Input: part model. Units: mm. Frame: model coordinates. A direction names the side the tool comes from. Round coordinates to 2 decimals unless told otherwise and drop trailing zeros. Loops run counter-clockwise (first coordinate to the right, second up) from the corner with the lowest first, then second, coordinate; pieces in that order, holes last. Notation, with made-up numbers: M 49,-13.5 L 73,-13.5 A25 cw 73,-1.5 Z; hole C -8.75,-31.75 d8. An arc over 180 degrees is marked long. Return JSON: item names as keys, results as strings. Group by question number.
1) Contact query for flat-ended pins moving along their axis: P1, Ø4, axis at x = 79, y = -17, coming from the +Z side; P2, Ø9, axis at x = -4.5, y = -15.5, coming from the -Z side; P3, Ø6.5, axis at x = -4.5, y = -19.5, coming from the +Z side; P4, Ø9.5, axis at y = -16.5, z = 15, coming from the +X side. Output: stop coordinate, or through.
2) Access query for faces 1 (the face through (12.5, -12, 71)), 2 (the face through (21, -12, -17)), 3 (the face through (21, -19.3, -2.5)), 4 (the face through (-21, -12, 17)). Directions: +Z, -Z, +X, -X, +Y, -Y. A direction counts if a zero-diameter tool reaches every point of the face in a straight line with its end or side. Return the directions, or none.
3) Section A-A (x = 0). Count the separate pieces of the cut face and the enclosed holes in it, plus the area to 3 significant figures.
4) Material intervals for line 1 (Z direction, x = 19.45, y = -14.5); line 2 (X direction, y = -18, z = 77); line 3 (Z direction, x = 122.65, y = -14.5), sorted ascending. Write a range as from..to.
5) Mould query, pull axis Z, two halves, no side actions, for faces 5 (the face through (1.08, -9.62, -18.46)), 6 (the face through (-73, -12, -12.5)), 7 (the face through (16, -20, 0)). Classes: +Z half, -Z half, draft (parallel to the pull), parting line (faces both ways), or undercut.
6) Section C-C (z = 82). Output: boundary loops of the cut face in (x, y), plus the area to 3 significant figures.
from build123d import *

# Parameters (mm, degrees)
F0_W      = 42
F0_H      = 42
F0_W_2    = 32
F0_H_2    = 32
F5_DEPTH  = 25
F1_W      = 25
F1_H      = 102
F2_W      = 102
F2_H      = 25
F3_W      = 102
F3_H      = 25
F4_W      = 25
F4_H      = 102
F6_DEPTH  = 25
F7_W      = 32
F7_H      = 32
F8_DEPTH  = 18
F9_W      = 100
F9_H      = 21
F10_DEPTH = 21
F11_W     = 100
F11_H     = 21
F12_DEPTH = 21
F13_W     = 21
F13_H     = 100
F14_DEPTH = 21
F15_W     = 21
F15_H     = 100
F16_DEPTH = 21
F18_D     = 10
F18_DEPTH = 11
F20_D     = 10
F20_DEPTH = 11
F22_D     = 10
F22_DEPTH = 11
F24_D     = 10
F24_DEPTH = 11
F26_D     = 20.9
F26_DEPTH = 3
F28_D     = 20.9
F28_DEPTH = 3
F30_D     = 20.9
F30_DEPTH = 3
F32_D     = 20.9
F32_DEPTH = 3


with BuildPart() as f5:
    # F0 (on Front) → F5 (new body)
    with BuildSketch(Plane.XZ):
        Rectangle(F0_W, F0_H)
        Rectangle(F0_W_2, F0_H_2, mode=Mode.SUBTRACT)
        Rectangle(F0_W_2, F0_H_2)
    extrude(amount=F5_DEPTH)

    # F1 (on Front) + F2 (on Front) + F3 (on Front) + F4 (on Front) → F6 (join)
    with BuildSketch(Plane.XZ):
        with Locations((0, -72)):
            Rectangle(F1_W, F1_H)
    with BuildSketch(Plane.XZ):
        with Locations((-72, 0)):
            Rectangle(F2_W, F2_H)
    with BuildSketch(Plane.XZ):
        with Locations((72, 0)):
            Rectangle(F3_W, F3_H)
    with BuildSketch(Plane.XZ):
        with Locations((0, 72)):
            Rectangle(F4_W, F4_H)
    extrude(amount=F6_DEPTH)

    # F7 (on face) → F8 (cut)
    with BuildSketch(Plane.XZ.offset(25)):
        Rectangle(F7_W, F7_H)
    extrude(amount=-F8_DEPTH, mode=Mode.SUBTRACT)

    # F9 (on face) → F10 (cut)
    with BuildSketch(Plane.XZ.offset(25)):
        with Locations((-71, 0)):
            Rectangle(F9_W, F9_H)
    extrude(amount=-F10_DEPTH, mode=Mode.SUBTRACT)

    # F11 (on face) → F12 (cut)
    with BuildSketch(Plane.XZ.offset(25)):
        with Locations((71, 0)):
            Rectangle(F11_W, F11_H)
    extrude(amount=-F12_DEPTH, mode=Mode.SUBTRACT)

    # F13 (on face) → F14 (cut)
    with BuildSketch(Plane.XZ.offset(25)):
        with Locations((0, 71)):
            Rectangle(F13_W, F13_H)
    extrude(amount=-F14_DEPTH, mode=Mode.SUBTRACT)

    # F15 (on face) → F16 (cut)
    with BuildSketch(Plane.XZ.offset(25)):
        with Locations((0, -71)):
            Rectangle(F15_W, F15_H)
    extrude(amount=-F16_DEPTH, mode=Mode.SUBTRACT)

    # F18
    with Locations(Plane.YZ.offset(21)):
        with Locations((-14.5, 0)):
            Hole(F18_D / 2, depth=F18_DEPTH)

    # F20
    with Locations(Plane(origin=(0, 0, -21), x_dir=(1, 0, 0), z_dir=(0, 0, -1))):
        with Locations((0, 14.5)):
            Hole(F20_D / 2, depth=F20_DEPTH)

    # F22
    with Locations(Plane.XY.offset(21)):
        with Locations((0, -14.5)):
            Hole(F22_D / 2, depth=F22_DEPTH)

    # F24
    with Locations(Plane(origin=(-21, 0, 0), x_dir=(0, -1, 0), z_dir=(-1, 0, 0))):
        with Locations((14.5, 0)):
            Hole(F24_D / 2, depth=F24_DEPTH)

    # F26
    with Locations(Plane(origin=(-123, 0, 0), x_dir=(0, -1, 0), z_dir=(-1, 0, 0))):
        with Locations((14.5, 0)):
            Hole(F26_D / 2, depth=F26_DEPTH)

    # F28
    with Locations(Plane.XY.offset(123)):
        with Locations((0, -14.5)):
            Hole(F28_D / 2, depth=F28_DEPTH)

    # F30
    with Locations(Plane(origin=(0, 0, -123), x_dir=(1, 0, 0), z_dir=(0, 0, -1))):
        with Locations((0, 14.5)):
            Hole(F30_D / 2, depth=F30_DEPTH)

    # F32
    with Locations(Plane.YZ.offset(123)):
        with Locations((-14.5, 0)):
            Hole(F32_D / 2, depth=F32_DEPTH)


solid = f5.part
Returned:
{
 "1": {"P1": "stops at z = 12.5", "P2": "stops at z = -21", "P3": "stops at z = 21", "P4": "stops at x = 123"},
 "2": {"face 1": "+Z, +X, +Y, -Y", "face 2": "-Z, +X, +Y, -Y", "face 3": "-Y", "face 4": "+Z, -X, +Y, -Y"},
 "3": {"separate pieces": "5", "enclosed holes": "0", "area": "1,190 mm^2"},
 "4": {"line 1": "z = -21..-5, 5..21", "line 2": "x = -12.5..-10.5, 10.5..12.5", "line 3": "z = -12.5..-10.45, 10.45..12.5"},
 "5": {"face 5": "draft", "face 6": "-Z half", "face 7": "undercut"},
 "6": {"outline": "M -12.5,-25 L -10.5,-25 L -10.5,-4 L 10.5,-4 L 10.5,-25 L 12.5,-25 L 12.5,0 L -12.5,0 Z", "area": "184 mm^2"}
}
